```python
from build123d import *

# Parameters (mm, degrees)
SKETCH_1_W           = 36.5
SKETCH_1_H           = 36.5
SKETCH_1_R           = 5.5
EXTRUDE_1_DEPTH      = 5
EXTRUDE_START        = 5
SKETCH_1_18_W        = 36.5
SKETCH_1_18_H        = 36.5
SKETCH_1_18_W_2      = 28.5
SKETCH_1_18_H_2      = 28.5
EXTRUDE_2_DEPTH      = 10
SKETCH_2_R           = 1.5
CUT_EXTRUDE_1_DEPTH  = 52.122402134
SKETCH_2_3_R         = 2.25
CUT_EXTRUDE_2_DEPTH  = 2
CUT_EXTRUDE_START    = -34.5
SKETCH_2_4_R         = 2.25
SKETCH_2_4_R_2       = 1.5
CUT_EXTRUDE_3_DEPTH  = 2
SKETCH_3_R           = 1.5
CUT_EXTRUDE_4_DEPTH  = 44.477724181
SKETCH_3_4_R         = 2.25
CUT_EXTRUDE_8_DEPTH  = 2
SKETCH_3_5_R         = 2.25
CUT_EXTRUDE_9_DEPTH  = 2
EXTRUDE_START_2      = 6
SKETCH_4_W           = 32.5
SKETCH_4_H           = 22
SKETCH_4_R           = 5.5
EXTRUDE_3_DEPTH      = 6
EXTRUDE_START_3      = 14
SKETCH_4_3_W         = 32.5
SKETCH_4_3_H         = 22
EXTRUDE_4_DEPTH      = 8
CUT_EXTRUDE_START_2  = 6
SKETCH_4_4_R         = 1
CUT_EXTRUDE_10_DEPTH = 5
EXTRUDE_5_DEPTH      = 2
SKETCH_4_6_R         = 0.75
CUT_EXTRUDE_11_DEPTH = 4
CUT_EXTRUDE_12_REACH = 48.24
SKETCH_4_7_R         = 1.5
SKETCH_5_W           = 200
SKETCH_5_H           = 100
CUT_EXTRUDE_13_DEPTH = 47.239863754


with BuildPart() as part:
    # 草图1 → 凸台-拉伸1 (new body)
    with BuildSketch(Plane(origin=(0, 0, 0), x_dir=(1, 0, 0), z_dir=(0, 1, 0))):
        with Locations((14.25, 0)):
            Rectangle(SKETCH_1_W, SKETCH_1_H)
        with Locations(Location((14.25, 0, 0), (0, 0, 270))):
            Circle(SKETCH_1_R, mode=Mode.SUBTRACT)
    extrude(amount=EXTRUDE_1_DEPTH)

    # 草图1<18> → 凸台-拉伸2 (add)
    with BuildSketch(Plane(origin=(0, 0, 0), x_dir=(1, 0, 0), z_dir=(0, 1, 0)).offset(EXTRUDE_START)):
        with Locations((14.25, 0)):
            Rectangle(SKETCH_1_18_W, SKETCH_1_18_H)
        with Locations((14.25, 0)):
            Rectangle(SKETCH_1_18_W_2, SKETCH_1_18_H_2, mode=Mode.SUBTRACT)
    extrude(amount=EXTRUDE_2_DEPTH)

    # 草图2 → 切除-拉伸1 (cut, through all)
    with BuildSketch(Plane(origin=(0, 0, -18.25), x_dir=(-1, 0, 0), z_dir=(0, 0, -1))):
        with Locations((-23.15, 7.5)):
            Circle(SKETCH_2_R)
        with Locations((-5.35, 7.5)):
            Circle(SKETCH_2_R)
    extrude(amount=-CUT_EXTRUDE_1_DEPTH, mode=Mode.SUBTRACT)

    # 草图2<3> → 切除-拉伸2 (cut)
    with BuildSketch(Plane(origin=(0, 0, -18.25), x_dir=(-1, 0, 0), z_dir=(0, 0, -1))):
        with Locations((-23.15, 7.5)):
            Circle(SKETCH_2_3_R)
        with Locations((-5.35, 7.5)):
            Circle(SKETCH_2_3_R)
    extrude(amount=-CUT_EXTRUDE_2_DEPTH, mode=Mode.SUBTRACT)

    # 草图2<4> → 切除-拉伸3 (cut)
    # profile 1 of 2: a face of its own
    with BuildSketch(Plane(origin=(0, 0, -18.25), x_dir=(-1, 0, 0), z_dir=(0, 0, -1)).offset(CUT_EXTRUDE_START)):
        with Locations((-23.15, 7.5)):
            Circle(SKETCH_2_4_R)
        with Locations(Location((-23.15, 7.5, 0), (0, 0, 180))):
            Circle(SKETCH_2_4_R_2, mode=Mode.SUBTRACT)
    # profile 2 of 2: a face of its own
    with BuildSketch(Plane(origin=(0, 0, -18.25), x_dir=(-1, 0, 0), z_dir=(0, 0, -1)).offset(CUT_EXTRUDE_START)):
        with Locations((-5.35, 7.5)):
            Circle(SKETCH_2_4_R)
        with Locations(Location((-5.35, 7.5, 0), (0, 0, 180))):
            Circle(SKETCH_2_4_R_2, mode=Mode.SUBTRACT)
    extrude(amount=-CUT_EXTRUDE_3_DEPTH, mode=Mode.SUBTRACT)

    # 草图3 → 切除-拉伸4 (cut, through all)
    with BuildSketch(Plane.ZY.offset(4)):
        with Locations((-8.9, 7.5)):
            Circle(SKETCH_3_R)
        with Locations((8.9, 7.5)):
            Circle(SKETCH_3_R)
    extrude(amount=-CUT_EXTRUDE_4_DEPTH, mode=Mode.SUBTRACT)

    # 草图3<4> → 切除-拉伸8 (cut)
    with BuildSketch(Plane.ZY.offset(4)):
        with Locations((-8.9, 7.5)):
            Circle(SKETCH_3_4_R)
        with Locations((8.9, 7.5)):
            Circle(SKETCH_3_4_R)
    extrude(amount=-CUT_EXTRUDE_8_DEPTH, mode=Mode.SUBTRACT)

    # 草图3<5> → 切除-拉伸9 (cut)
    with BuildSketch(Plane.ZY.offset(4).offset(CUT_EXTRUDE_START)):
        with Locations((-8.9, 7.5)):
            Circle(SKETCH_3_5_R)
        with Locations((8.9, 7.5)):
            Circle(SKETCH_3_5_R)
    extrude(amount=-CUT_EXTRUDE_9_DEPTH, mode=Mode.SUBTRACT)

    # 草图4 → 凸台-拉伸3 (add)
    with BuildSketch(Plane.XZ.offset(EXTRUDE_START_2)):
        with Locations((23.5, 0)):
            Rectangle(SKETCH_4_W, SKETCH_4_H)
        with Locations(Location((14.25, 0, 0), (0, 0, 270))):
            Circle(SKETCH_4_R, mode=Mode.SUBTRACT)
    extrude(amount=-EXTRUDE_3_DEPTH)

    # 草图4<3> → 凸台-拉伸4 (add)
    with BuildSketch(Plane.XZ.offset(EXTRUDE_START_3)):
        with Locations((23.5, 0)):
            Rectangle(SKETCH_4_3_W, SKETCH_4_3_H)
        with BuildLine():
            ThreePointArc((18.067307692, 3.959565883), (27.052586177, 9.998051199), (36.269230769, 4.318967044))
            ThreePointArc((36.269230769, 4.318967044), (38.08567491, 2.490366053), (38.75, 0))
            ThreePointArc((38.75, 0), (38.08567491, -2.490366053), (36.269230769, -4.318967044))
            ThreePointArc((36.269230769, -4.318967044), (27.052586177, -9.998051199), (18.067307692, -3.959565883))
            ThreePointArc((18.067307692, -3.959565883), (8.75, 0), (18.067307692, 3.959565883))
        make_face(mode=Mode.SUBTRACT)
    extrude(amount=-EXTRUDE_4_DEPTH)

    # 草图4<4> → 切除-拉伸10 (cut)
    with BuildSketch(Plane.XZ.offset(CUT_EXTRUDE_START_2)):
        with Locations(Location((27.25, 0, 0), (0, 0, 270))):
            Circle(SKETCH_4_4_R)
    extrude(amount=-CUT_EXTRUDE_10_DEPTH, mode=Mode.SUBTRACT)

    # 草图4<5> → 凸台-拉伸5 (add)
    with BuildSketch(Plane.XZ):
        Polygon((39.75, 11), (39.75, 15.5), (2.75, 15.5), (2.75, -15.5), (39.75, -15.5), (39.75, -11), (7.25, -11), (7.25, 11), align=None)
    extrude(amount=EXTRUDE_5_DEPTH)

    # 草图4<6> → 切除-拉伸11 (cut)
    with BuildSketch(Plane.XZ):
        with Locations(Location((23.5, 13.25, 0), (0, 0, 90))):
            Circle(SKETCH_4_6_R)
        with Locations(Location((5, 0, 0), (0, 0, 90))):
            Circle(SKETCH_4_6_R)
        with Locations(Location((23.5, -13.25, 0), (0, 0, 90))):
            Circle(SKETCH_4_6_R)
    extrude(amount=-CUT_EXTRUDE_11_DEPTH, mode=Mode.SUBTRACT)

    # 草图4<7> → 切除-拉伸12 (cut, up to next)
    with BuildSketch(Plane.XZ, mode=Mode.PRIVATE) as cut_extrude_12_sk1:
        with Locations(Location((23.5, 13.25, 0), (0, 0, 90))):
            Circle(SKETCH_4_7_R)
    cut_extrude_12_tool1 = extrude(cut_extrude_12_sk1.sketch, amount=CUT_EXTRUDE_12_REACH, mode=Mode.PRIVATE) & part.part
    # 草图4<7> → 切除-拉伸12 (cut, up to next)
    with BuildSketch(Plane.XZ, mode=Mode.PRIVATE) as cut_extrude_12_sk2:
        with Locations(Location((5, 0, 0), (0, 0, 90))):
            Circle(SKETCH_4_7_R)
    cut_extrude_12_tool2 = extrude(cut_extrude_12_sk2.sketch, amount=CUT_EXTRUDE_12_REACH, mode=Mode.PRIVATE) & part.part
    # 草图4<7> → 切除-拉伸12 (cut, up to next)
    with BuildSketch(Plane.XZ, mode=Mode.PRIVATE) as cut_extrude_12_sk3:
        with Locations(Location((23.5, -13.25, 0), (0, 0, 90))):
            Circle(SKETCH_4_7_R)
    cut_extrude_12_tool3 = extrude(cut_extrude_12_sk3.sketch, amount=CUT_EXTRUDE_12_REACH, mode=Mode.PRIVATE) & part.part
    add(cut_extrude_12_tool1.solids().sort_by_distance((23.5, 0, 13.25))[0], mode=Mode.SUBTRACT)
    add(cut_extrude_12_tool2.solids().sort_by_distance((5, 0, 0))[0], mode=Mode.SUBTRACT)
    add(cut_extrude_12_tool3.solids().sort_by_distance((23.5, 0, -13.25))[0], mode=Mode.SUBTRACT)

    # 草图5 → 切除-拉伸13 (cut, through all)
    with BuildSketch(Plane.XZ):
        Rectangle(SKETCH_5_W, SKETCH_5_H)
    extrude(amount=CUT_EXTRUDE_13_DEPTH, mode=Mode.SUBTRACT)


solid = part.part
```
Read the model definition and answer for the solid it produces. Units are mm, in the model's axes. A direction names the side the tool comes from. Give positions to 0.01 mm unless a question says otherwise; leave off trailing zeros. Loops run counter-clockwise (first coordinate to the right, second up) from the corner with the lowest first, then second, coordinate; pieces in that order, holes last.
Item 1: The part is cut by section B-B (x = 14.25). Write down the section's boundary in (y, z).
Item 2: Each of these flat-tipped pins is pushed along its axis until it touches: pin 1 Ø1.4 at (x, z) = (5, 0) entering from +Y; pin 2 Ø3.5 at (x, y) = (5.35, 7.5) entering from -Z; pin 3 Ø3.5 at (x, y) = (5.35, 7.5) entering from +Z. Where does it stop, or does it pass through?
Item 3: The part is cut by section D-D (x = 0.5). Write down the section's boundary in (y, z).
Item 4: Find the intervals of material crossed by line 1 along X through (y, z) = (14.25, -11.5); line 2 along Z through (x, y) = (11, 10.25); line 3 along Y through (x, z) = (20, 10), in increasing order.
Item 5: The part is cut by section A-A (z = 0). Write down the section's boundary in (x, y), and give its area (4 significant figures).
Item 6: The part is cut by section C-C (y = 10.5). Write down the section's boundary in (x, z), and give its area (3 significant figures).
Item 7: The mould has two halves that part along X. Classify faces 5 (the flat face through (-2, 6, -8)), 6 (the cylindrical face through (4.14, 9.397, 17.236)), 7 (the flat face through (24, 6, 16.25)), 8 (the cylindrical face through (31.49, 9.02, 7.24)): released by +X, released by -X, zero draft, split by the parting line, or undercut.
Item 8: For faces 1 (the cylindrical face through (-3.01, 9.02, 7.24)), 2 (the flat face through (30.5, 6, -8)), 3 (the cylindrical face through (21.004, 8.176, 17.236)), 4 (the flat face through (14, 10, 14.25)), determine the directions among +Z, -Z, +X, -X, +Y, -Y from which every point of the face is accessible in a straight line to the end or side of a thin tool.
Taken from the geometry:
1. outline: (0, -18.25) - (15, -18.25) - (15, -14.25) - (5, -14.25) - (5, -5.5) - (0, -5.5) - close; (0, 5.5) - (5, 5.5) - (5, 14.25) - (15, 14.25) - (15, 18.25) - (0, 18.25) - close
2. pin 1: stops at y = 5
2. pin 2: stops at z = -16.25
2. pin 3: stops at z = 16.25
3. outline: (0, -18.25) - (15, -18.25) - (15, -14.25) - (5, -14.25) - (5, 14.25) - (15, 14.25) - (15, 18.25) - (0, 18.25) - close
4. line 1: x = -4 to 0, 28.5 to 32.5
4. line 2: z = -18.25 to -14.25, 14.25 to 18.25
4. line 3: y = 0 to 5
5. outline: (-4, 0) - (4.25, 0) - (4.25, 4) - (5.75, 4) - (5.75, 0) - (8.75, 0) - (8.75, 5) - (0, 5) - (0, 15) - (-4, 15) - close; (19.75, 0) - (32.5, 0) - (32.5, 15) - (28.5, 15) - (28.5, 5) - (19.75, 5) - close
5. area: 201.5 mm2
6. outline: (-4, -18.25) - (32.5, -18.25) - (32.5, 18.25) - (-4, 18.25) - close; hole (0, -14.25) - (28.5, -14.25) - (28.5, 14.25) - (0, 14.25) - close
6. area: 520 mm2
7. face 5: released by -X
7. face 6: undercut
7. face 7: undercut
7. face 8: zero draft
8. face 1: -X
8. face 2: +X
8. face 3: +Z
8. face 4: +Y
